CAD build for the part. Positions are in the model's coordinates, mm. Round coordinates to 2 decimals unless told otherwise and drop trailing zeros. Order: outer loops, then holes, each group sorted by start corner. A loop starts at its lowest first (then second) coordinate and runs counter-clockwise, first axis right, second up. Notation, with made-up numbers: (4, 83) -> (57, 83) arc R7 ccw to (57, 95) -> close; hole circle Ø11 at (20, 46). An arc over 180 degrees is marked (long way). Return JSON: item names as keys, results as strings. Group by question number.
Q1. Cut at A-A (y = 6). Write the cut outline in (x, z), then the cut area to 3 significant figures.
Q2. Cut at B-B (z = 1.25). Count the separate pieces of the cut face and the enclosed holes in it, then the cut area to 3 significant figures.
Q3. Flat gauge pins, fed straight in: pin 1 (0.8 mm diameter, centred on y = -1.5, z = 2, fed in from -X); pin 2 (1.5 mm diameter, centred on x = 56, z = 2.5, fed in from -Y). Where does each tip first touch, or does it go through?
Q4. Cut at C-C (x = 19.5). Write the cut outline in (y, z), then the cut area to 3 significant figures.
Q5. Probe line 1 along X through (y, z) = (18.5, 2.05); line 2 along X through (y, z) = (3.5, 0.5); line 3 along Y through (x, z) = (9.5, 1.2). List the from-to ranges inside material, lowest first.
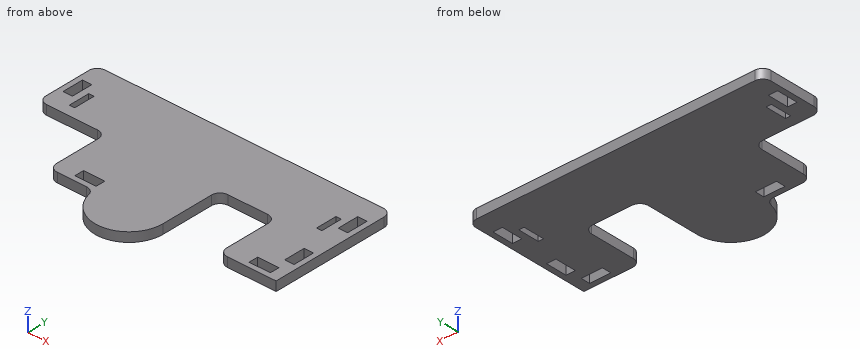
from build123d import *

# Parameters (mm, degrees)
BOSS_EXTRUDE1_DEPTH = 2.794
SKETCH3_W           = 2.794
SKETCH3_H           = 6.35
SKETCH3_W_2         = 1.5875
SKETCH3_W_3         = 6.35
SKETCH3_H_2         = 2.794
CUT_EXTRUDE1_DEPTH  = 78.110446656
FILLET1_R           = 2.54


with BuildPart() as part:
    # Sketch1 → Boss-Extrude1 (new body)
    with BuildSketch(Plane.XY):
        with BuildLine():
            Line((69.475359958, -4.3815), (69.475359958, 33.3375))
            Line((69.475359958, 33.3375), (-18.662640042, 33.3375))
            Line((-18.662640042, 33.3375), (-18.662640042, 14.2875))
            Line((-18.662640042, 14.2875), (1.5875, 14.2875))
            Line((1.5875, 14.2875), (1.5875, -4.3815))
            Line((1.5875, -4.3815), (15.094335312, -4.3815))
            ThreePointArc((15.094335312, -4.3815), (25.406359958, -14.226588915), (35.409491259, -4.0678))
            Line((35.409491259, -4.0678), (35.409491259, 14.2875))
            Line((35.409491259, 14.2875), (52.393859958, 14.2875))
            Line((52.393859958, 14.2875), (52.393859958, -4.3815))
            Line((52.393859958, -4.3815), (69.475359958, -4.3815))
        make_face()
    extrude(amount=BOSS_EXTRUDE1_DEPTH)

    # Sketch3 → Cut-Extrude1 (cut, through all)
    with BuildSketch(Plane.XY.offset(2.794)):
        with Locations((-15.678140042, 23.8125)):
            Rectangle(SKETCH3_W, SKETCH3_H)
        with Locations((66.490859958, 23.8125)):
            Rectangle(SKETCH3_W, SKETCH3_H)
        with Locations((66.490859958, 6.35)):
            Rectangle(SKETCH3_W, SKETCH3_H)
        with Locations((-11.518890042, 20.6375)):
            Rectangle(SKETCH3_W_2, SKETCH3_H)
        with Locations((62.331609958, 20.6375)):
            Rectangle(SKETCH3_W_2, SKETCH3_H)
        with Locations((11.1125, -1.397)):
            Rectangle(SKETCH3_W_3, SKETCH3_H_2)
        with Locations((63.125359958, -1.397)):
            Rectangle(SKETCH3_W_3, SKETCH3_H_2)
    extrude(amount=-CUT_EXTRUDE1_DEPTH, mode=Mode.SUBTRACT)

    # Fillet1
    fillet1_edges = [part.edges().sort_by_distance(p)[0] for p in [
        (52.393859958, -4.3815, 1.397),
        (52.393859958, 14.2875, 1.397),
        (35.409491259, 14.2875, 1.397),
        (15.094335312, -4.3815, 1.397),
        (1.5875, -4.3815, 1.397),
        (1.5875, 14.2875, 1.397),
        (-18.662640042, 14.2875, 1.397),
        (-18.662640042, 33.3375, 1.397),
        (69.475359958, 33.3375, 1.397),
    ]]
    fillet(fillet1_edges, radius=FILLET1_R)


solid = part.part
Solution:
{
 "1": {"outline": "(1.59, 0) -> (35.41, 0) -> (35.41, 2.79) -> (1.59, 2.79) -> close; (52.39, 0) -> (65.09, 0) -> (65.09, 2.79) -> (52.39, 2.79) -> close; (67.89, 0) -> (69.48, 0) -> (69.48, 2.79) -> (67.89, 2.79) -> close", "area": "134 mm²"},
 "2": {"separate pieces": "1", "enclosed holes": "7", "area": "2,670 mm²"},
 "3": {"pin 1": "stops at x = 1.59", "pin 2": "stops at y = -4.38"},
 "4": {"outline": "(-12.44, 0) -> (33.34, 0) -> (33.34, 2.79) -> (-12.44, 2.79) -> close", "area": "128 mm²"},
 "5": {"line 1": "x = -18.66 to -12.31, -10.73 to 61.54, 63.13 to 69.48", "line 2": "x = 1.59 to 35.41, 52.39 to 65.09, 67.89 to 69.48", "line 3": "y = -4.38 to -2.79, 0 to 33.34"}
}
